```python
from build123d import *

# Parameters (mm, degrees)
BOSS_EXTRUDE1_DEPTH              = 44.45
F_1_4_0_25_DIAMETER_HOLE2_D      = 6.35
FILLET1_R                        = 9.525
F_13_64_0_20313_DIAMETER_HOLE1_D = 5.159375


with BuildPart() as part:
    # Sketch1 → Boss-Extrude1 (new body)
    with BuildSketch(Plane.XY):
        Polygon((0, 0), (0, 25.4), (3.175, 25.4), (3.175, 3.175), (25.4, 3.175), (25.4, 0), align=None)
    extrude(amount=BOSS_EXTRUDE1_DEPTH)

    # 1/4 (0.25) Diameter Hole2 (through all)
    with Locations(Plane.ZY):
        with Locations((22.225, 17.4625)):
            Hole(F_1_4_0_25_DIAMETER_HOLE2_D / 2)

    # Fillet1
    fillet1_edges = [part.edges().sort_by_distance(p)[0] for p in [
        (1.5875, 25.4, 44.45),
        (1.5875, 25.4, 0),
    ]]
    fillet(fillet1_edges, radius=FILLET1_R)

    # 13/64 (0.20313) Diameter Hole1 (through all)
    with Locations(Plane(origin=(0, 0, 0), x_dir=(-1, 0, 0), z_dir=(0, -1, 0))):
        with Locations((-12.7, -38.1), (-12.7, -6.35)):
            Hole(F_13_64_0_20313_DIAMETER_HOLE1_D / 2)


solid = part.part
```
Part model, mm, in its own coordinate system. A direction names the side the tool comes from. Coordinates: 2 decimals unless noted, no trailing zeros. Loops run counter-clockwise (first coordinate to the right, second up) from the corner with the lowest first, then second, coordinate; pieces in that order, holes last. Notation, with made-up numbers: (70.25, 64.25) - (123.25, 64.25) arc R36 ccw to (123.25, 99.25) - close; hole circle Ø9 at (35, 69). An arc over 180 degrees is marked (long way). Write item = value, one per line. Start each with the question number.
Item 1: 3-axis set-ups, long thin cutter, end or side, ignore diameter. For faces 4 (the flat face through (9, 3, 44.45)), 5 (the flat face through (14, 3.175, 22)): which of +Z, -Z, +X, -X, +Y, -Y reach the whole face in a straight line?
Item 2: Mould opens along Z. For faces 1 (the cylindrical face through (1.61, 18.416, 19.197)), 2 (the flat face through (25.4, 2, 22)), 3 (the flat face through (9, 3, 0)) say: released by +Z, released by -Z, zero draft, split by the parting line, or undercut.
Item 3: Cut at A-A, the plane x = 12.7. Give the cut face in (y, z) (3 decimals), and give its area (3 significant figures).
Item 4: Cut at B-B, the plane y = 19. Give the cut face in (x, z) (3 decimals).
Item 5: Flat gauge pins, fed straight in: pin 1 Ø1 at (y, z) = (13.5, 13.5) entering from -X; pin 2 Ø6.5 at (x, z) = (18.5, 15.5) entering from +Y (3 decimals). Where does each tip first touch, or does it go through?
Item 6: Cut at D-D, the plane z = 32. Give the cut face in (x, y) (3 decimals), and give its area (3 significant figures).
Item 7: Cut at C-C, the plane z = 38.1. Give the cut face in (x, y) (3 decimals).
Item 8: Wall check: L1, parallel to X at y = 1.8, z = 38.1; L2, parallel to Z at x = 12.7, y = 0.95; L3, parallel to Y at x = 24.75, z = 8.5 (3 decimals). Give the ranges that are in metal, low to high. Write a range as from..to.
The answers:
q1.face_4 = +Z, +X, -X, +Y, -Y
q1.face_5 = +Z, -Z, +X, +Y
q2.face_1 = undercut
q2.face_2 = zero draft
q2.face_3 = released by -Z
q3.outline = (0, 0) - (3.175, 0) - (3.175, 3.77) - (0, 3.77) - close; (0, 8.93) - (3.175, 8.93) - (3.175, 35.52) - (0, 35.52) - close; (0, 40.68) - (3.175, 40.68) - (3.175, 44.45) - (0, 44.45) - close
q3.area = 108 mm2
q4.outline = (0, 0.527) - (3.175, 0.527) - (3.175, 19.447) - (0, 19.447) - close; (0, 25.003) - (3.175, 25.003) - (3.175, 43.923) - (0, 43.923) - close
q5.pin_1 = 0
q5.pin_2 = 3.175
q6.outline = (0, 0) - (25.4, 0) - (25.4, 3.175) - (3.175, 3.175) - (3.175, 25.4) - (0, 25.4) - close
q6.area = 151 mm2
q7.outline = (0, 0) - (10.12, 0) - (10.12, 3.175) - (3.175, 3.175) - (3.175, 24.855) - (0, 24.855) - close; (15.28, 0) - (25.4, 0) - (25.4, 3.175) - (15.28, 3.175) - close
q8.L1 = 0..10.12, 15.28..25.4
q8.L2 = 0..3.77, 8.93..35.52, 40.68..44.45
q8.L3 = 0..3.175
